```python
from build123d import *

# Parameters (mm, degrees)
SKETCH1_W           = 70
SKETCH1_H           = 50
SKETCH1_R           = 2
SKETCH1_R_2         = 6.5
BOSS_EXTRUDE1_DEPTH = 9
SKETCH5_R           = 2.1
CUT_EXTRUDE1_DEPTH  = 9
SKETCH6_R           = 3.25
CUT_EXTRUDE2_DEPTH  = 3
FILLET1_R           = 2
BOSS_EXTRUDE3_START = -4.5
SKETCH8_R           = 6.5
BOSS_EXTRUDE3_DEPTH = 4.5


with BuildPart() as part:
    # Sketch1 → Boss-Extrude1 (new body)
    with BuildSketch(Plane(origin=(0, 0, 0), x_dir=(1, 0, 0), z_dir=(0, 1, 0))):
        with Locations((-28.500824125, 0.1029652)):
            Rectangle(SKETCH1_W, SKETCH1_H)
        with Locations(Location((-58.528775182, 20.1029652, 0), (0, 0, 270))):
            Circle(SKETCH1_R, mode=Mode.SUBTRACT)
        with Locations(Location((-58.500824125, -19.8970348, 0), (0, 0, 270))):
            Circle(SKETCH1_R, mode=Mode.SUBTRACT)
        with Locations(Location((1.600142136, -19.83023128, 0), (0, 0, 270))):
            Circle(SKETCH1_R, mode=Mode.SUBTRACT)
        with Locations(Location((1.499175875, 20.1029652, 0), (0, 0, 270))):
            Circle(SKETCH1_R, mode=Mode.SUBTRACT)
        with Locations(Location((-28.500824125, 0.1029652, 0), (0, 0, 270))):
            Circle(SKETCH1_R_2, mode=Mode.SUBTRACT)
    extrude(amount=BOSS_EXTRUDE1_DEPTH)

    # Sketch5 → Cut-Extrude1 (cut)
    with BuildSketch(Plane(origin=(0, 9, 0), x_dir=(1, 0, 0), z_dir=(0, 1, 0))):
        with Locations(Location((-35.4063316, 7.028451935, 0), (0, 0, 270))):
            Circle(SKETCH5_R)
        with Locations(Location((-21.595316651, -6.822521536, 0), (0, 0, 270))):
            Circle(SKETCH5_R)
    extrude(amount=-CUT_EXTRUDE1_DEPTH, mode=Mode.SUBTRACT)

    # Sketch6 → Cut-Extrude2 (cut)
    with BuildSketch(Plane(origin=(0, 9, 0), x_dir=(1, 0, 0), z_dir=(0, 1, 0))):
        with Locations(Location((-35.4063316, 7.028451935, 0), (0, 0, 270))):
            Circle(SKETCH6_R)
        with Locations(Location((-21.595316651, -6.822521536, 0), (0, 0, 270))):
            Circle(SKETCH6_R)
    extrude(amount=-CUT_EXTRUDE2_DEPTH, mode=Mode.SUBTRACT)

    # Fillet1
    fillet1_edges = [part.edges().sort_by_distance(p)[0] for p in [
        (6.499175875, 4.5, -25.1029652),
        (6.499175875, 4.5, 24.8970348),
        (-63.500824125, 4.5, 24.8970348),
        (-63.500824125, 4.5, -25.1029652),
    ]]
    fillet(fillet1_edges, radius=FILLET1_R)

    # Sketch8 → Boss-Extrude3 (add)
    with BuildSketch(Plane(origin=(0, 9, 0), x_dir=(1, 0, 0), z_dir=(0, 1, 0)).offset(BOSS_EXTRUDE3_START)):
        with Locations(Location((-28.500824125, 0.1029652, 0), (0, 0, 270))):
            Circle(SKETCH8_R)
    extrude(amount=BOSS_EXTRUDE3_DEPTH)


solid = part.part
```
Geometry: final body of the model. Coordinates: model frame, mm. A direction names the side the tool comes from. Give positions to 0.01 mm unless a question says otherwise; leave off trailing zeros. Loops run counter-clockwise (first coordinate to the right, second up) from the corner with the lowest first, then second, coordinate; pieces in that order, holes last. Notation, with made-up numbers: (-22.75, -18.75) - (32.25, -18.75) arc R10 ccw to (32.25, -0.75) - close; hole circle Ø9 at (-10, 57). An arc over 180 degrees is marked (long way). Answer as CSV lines item,"result". Start each with the question number.
(1) Pin query (flat end, axial travel): P1, Ø21, axis at x = -28.5, z = -0.1, coming from the -Y side; P2, Ø3.5, axis at x = 1.6, z = 19.83, coming from the +Y side; P3, Ø4, axis at x = -27.5, z = 0.5, coming from the -Y side; P4, Ø6, axis at x = -21.6, z = 6.82, coming from the +Y side. Return the tip coordinate at first contact, or that it passes through.
(2) Section query B-B (y = 3). Output: boundary loops of the cut face in (x, z).
(3) Section query D-D (z = -1.5). Output: boundary loops of the cut face in (x, y).
(4) Ray query, line 1 along X through (y, z) = (4, -7); line 2 along X through (y, z) = (0.5, 19.5); line 3 along Z through (x, y) = (-58, 6.5). Return the intervals inside material, ascending. Write a range as [from, to].
(5) Section query A-A (z = -21). Output: boundary loops of the cut face in (x, y), and give its area (3 significant figures).
(6) Reachability of faces 4 (the face through (0.834, 4.437, 21.678)), 5 (the face through (-18.855, 7.521, 8.57)), 6 (the face through (-34.846, 2.218, -1.512)) from +Z, -Z, +X, -X, +Y, -Y: full face, straight path, thin tool, end or side. Return the list, or none.
(7) Mould query, pull axis Y, two halves, no side actions, for faces 1 (the face through (-60.303, 4.437, -19.18)), 2 (the face through (-28, 4.5, 0)), 3 (the face through (-38, 6, -7)). Classes: +Y half, -Y half, draft (parallel to the pull), parting line (faces both ways), or undercut.
(8) Section query C-C (x = 0.5). Output: boundary loops of the cut face in (y, z).
Worked answers:
1,P1,"stops at y = 0"
1,P2,"passes through"
1,P3,"stops at y = 4.5"
1,P4,"stops at y = 6"
2,outline,"(-63.5, -23.1) arc R2 ccw to (-61.5, -25.1) - (4.5, -25.1) arc R2 ccw to (6.5, -23.1) - (6.5, 22.9) arc R2 ccw to (4.5, 24.9) - (-61.5, 24.9) arc R2 ccw to (-63.5, 22.9) - close; hole circle Ø4 at (-58.53, -20.1); hole circle Ø4 at (-58.5, 19.9); hole circle Ø4.2 at (-35.41, -7.03); hole circle Ø13 at (-28.5, -0.1); hole circle Ø4.2 at (-21.6, 6.82); hole circle Ø4 at (1.5, -20.1); hole circle Ø4 at (1.6, 19.83)"
3,outline,"(-63.5, 0) - (-34.85, 0) - (-34.85, 4.5) - (-22.15, 4.5) - (-22.15, 0) - (6.5, 0) - (6.5, 9) - (-63.5, 9) - close"
4,line 1,"x = [-63.5, -37.51], [-33.31, 6.5]"
4,line 2,"x = [-63.5, -60.46], [-56.54, -0.37], [3.57, 6.5]"
4,line 3,"z = [-25.1, -22.03], [-18.17, 17.96], [21.83, 24.9]"
5,outline,"(-63.5, 0) - (-60.32, 0) - (-60.32, 9) - (-63.5, 9) - close; (-56.74, 0) - (-0.29, 0) - (-0.29, 9) - (-56.74, 9) - close; (3.29, 0) - (6.5, 0) - (6.5, 9) - (3.29, 9) - close"
5,area,"566 mm^2"
6,face 4,"+Y, -Y"
6,face 5,"+Y"
6,face 6,"-Y"
7,face 1,"draft"
7,face 2,"-Y half"
7,face 3,"+Y half"
8,outline,"(0, -25.1) - (9, -25.1) - (9, -21.84) - (0, -21.84) - close; (0, -18.37) - (9, -18.37) - (9, 18.16) - (0, 18.16) - close; (0, 21.5) - (9, 21.5) - (9, 24.9) - (0, 24.9) - close"
